from build123d import *

# Parameters (mm, degrees)
F0_R     = 12.5
F0_R_2   = 30
F1_DEPTH = 6
F2_R     = 20


with BuildPart() as f1:
    # F0 (on Front) → F1 (new body)
    with BuildSketch(Plane.XZ):
        with BuildLine():
            Line((17.497548, -33.390142), (35.297627, 0))
            ThreePointArc((35.297627, 0), (0, 58.816947), (-35.297627, 0))
            Line((-35.297627, 0), (-17.5, -33.683053))
            ThreePointArc((-17.5, -33.683053), (0.14646, -51.18244), (17.497548, -33.390142))
        make_face()
        with Locations((0, -33.683053)):
            Circle(F0_R, mode=Mode.SUBTRACT)
        with Locations((0, 18.816947)):
            Circle(F0_R_2, mode=Mode.SUBTRACT)
    extrude(amount=F1_DEPTH)

    # F2
    f2_edges = [f1.edges().sort_by_distance(p)[0] for p in [
        (17.497548, -3, -33.390142),
        (-17.5, -3, -33.683053),
    ]]
    fillet(f2_edges, radius=F2_R)


solid = f1.part
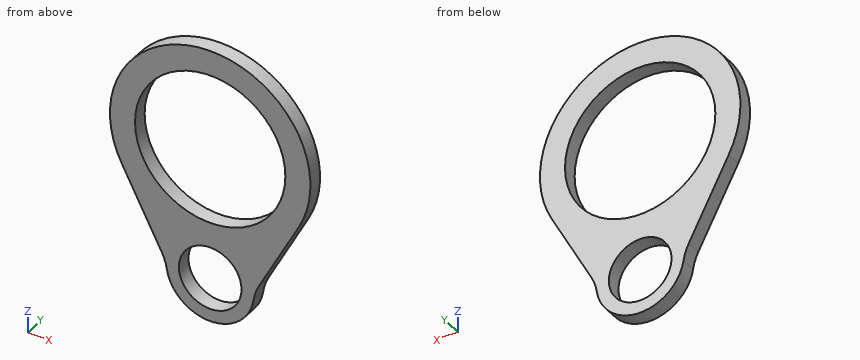
Design review of the part built by this model. Coordinates are the model's own, in mm. Give positions to 0.01 mm unless a question says otherwise; leave off trailing zeros. Loops run counter-clockwise (first coordinate to the right, second up) from the corner with the lowest first, then second, coordinate; pieces in that order, holes last. Notation, with made-up numbers: (-4, -25.5) - (12, -25.5) arc R25 ccw to (12, -1.5) - close; hole circle Ø11 at (75, 15.25). An arc over 180 degrees is marked (long way). Write item = value, one per line.
1) To check wall thickness, follow line 1 (Z direction, x = -3, y = -4.75); line 2 (Z direction, x = -11.5, y = -3.35); line 3 (Z direction, x = 19.5, y = -2.15). State the ranges of each line that lie inside material, in increasing order.
Result sheet:
line_1 = -50.92 to -45.82, -21.55 to -11.03, 48.67 to 58.7
line_2 = -46.87 to -38.58, -28.78 to -8.89, 46.53 to 57.13
line_3 = -29.63 to -3.98, 41.61 to 53.74
2) Take a section at A-A on x = 0. State the section outline as (y, z) points.
Result sheet:
outline = (-6, -51.18) - (0, -51.18) - (0, -46.18) - (-6, -46.18) - close; (-6, -21.18) - (0, -21.18) - (0, -11.18) - (-6, -11.18) - close; (-6, 48.82) - (0, 48.82) - (0, 58.82) - (-6, 58.82) - close
3) Take a section at C-C on y = -3. State the section outline as (x, z) points.
Result sheet:
outline = (-35.3, 0) - (-19.36, -30.16) arc R20 cw to (-17.29, -36.4) arc R17.5 ccw to (17.31, -36.22) arc R20 cw to (19.45, -29.72) - (35.3, 0) arc R40 ccw (long way) to start; hole circle Ø60 at (0, 18.82); hole circle Ø25 at (0, -33.68)
4) Clearance check with flat-ended pins moving along their axes: pin 1 Ø22.5 at (x, z) = (0, -33.68) entering from +Y; pin 2 Ø1.5 at (x, y) = (18.5, -3.5) entering from +Z; pin 3 Ø1.5 at (x, y) = (-26, -5.5) entering from +Z. State where each tip first meets the part, or that it passes through.
Result sheet:
pin_1 = through
pin_2 = 54.66
pin_3 = 49.84
5) Take a section at B-B on z = 14. State the section outline as (x, y) points.
Result sheet:
outline = (-39.71, -6) - (-29.61, -6) - (-29.61, 0) - (-39.71, 0) - close; (29.61, -6) - (39.71, -6) - (39.71, 0) - (29.61, 0) - close
6) Take a section at D-D on x = -8.5. State the section outline as (y, z) points.
Result sheet:
outline = (-6, -48.98) - (0, -48.98) - (0, -42.85) - (-6, -42.85) - close; (-6, -24.52) - (0, -24.52) - (0, -9.95) - (-6, -9.95) - close; (-6, 47.59) - (0, 47.59) - (0, 57.9) - (-6, 57.9) - close
